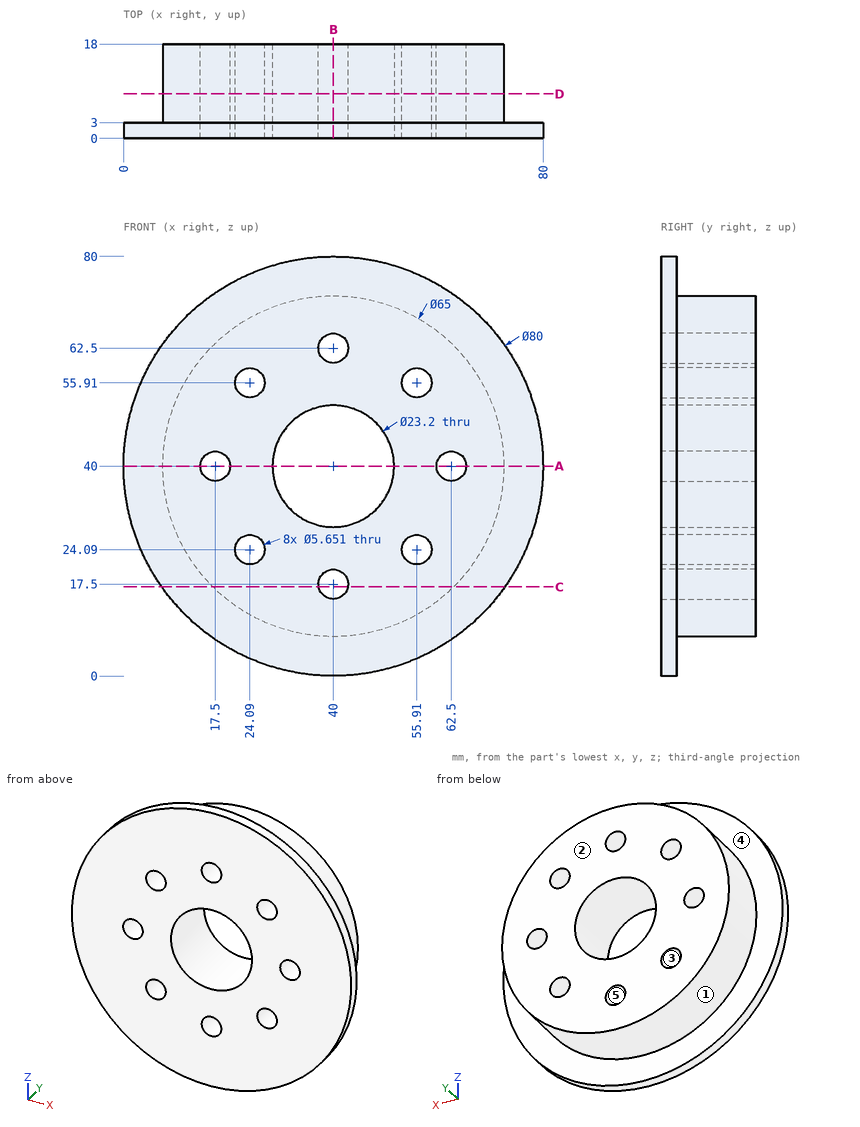
Here's the drawing with two shaded views (mm, measured from the low corner). I have some questions. A direction names the side the tool comes from. Give positions to 0.01 mm unless a question says otherwise; leave off trailing zeros. Write each loop counter-clockwise with the first axis right and the second up, starting at its lowest first coordinate (ties: lowest second). Pieces come first, ordered by that corner, then holes. Notation, with made-up numbers: (-9, 41) -> (13, 41) arc R27 cw to (13, 58) -> close; hole circle Ø4 at (27.5, 68.5). An arc over 180 degrees is marked (long way). Use one line per item in the form item = value. Start each with the question number.
1. Imagine slicing it at C-C on z = 17. List the corners of the cut face in (x, y) for me.
2. Imagine slicing it at D-D on y = 8.5. State how many separate pieces and enclosed holes the cut face has, plus the area to 4 significant figures.
3. Imagine slicing it at B-B on x = 40. List the corners of the cut face in (y, z) for me (1 decimal).
4. If I drill on L1, parallel to Z at x = 56.5, y = 3.25 (1 decimal); L2, parallel to X at y = 8.5, z = 22.5 (1 decimal), over which ranges is the centre line in solid material (lowest first)?
5. Will these pins go through, and if not, where does the flat tip stop? pin 1 Ø3 at (x, y) = (21.5, 9.5) entering from +Z; pin 2 Ø1.5 at (y, z) = (16, 65.5) entering from +X (1 decimal); pin 3 Ø10 at (x, y) = (52, 13.5) entering from -Z; pin 4 Ø4.5 at (x, z) = (55.91, 55.91) entering from -Y.
6. Imagine slicing it at A-A on z = 40. List the corners of the cut face in (x, y) for me (1 decimal), plus the area to 3 significant figures.
7. Thinking about a two-plate mould opening in Z: for the marked faces 1, 2 and 3, which applies, +Z half, -Z half, draft (parallel to the pull), parting line (faces both ways), or undercut?
8. On a 3-axis mill with a long thin cutter (end or side, diameter ignored), from which of +Z, -Z, +X, -X, +Y, -Y can I reach the whole of each face in a straight line? I mean the marked faces 4 and 5. Say none if no direction works.
Entries:
q1.outline = (7.27, 0) -> (37.22, 0) -> (37.22, 18) -> (17.04, 18) -> (17.04, 3) -> (7.27, 3) -> close; (42.78, 0) -> (72.73, 0) -> (72.73, 3) -> (62.96, 3) -> (62.96, 18) -> (42.78, 18) -> close
q2.separate_pieces = 1
q2.enclosed_holes = 9
q2.area = 2,695 mm²
q3.outline = (0, 0) -> (3, 0) -> (3, 7.5) -> (18, 7.5) -> (18, 14.7) -> (0, 14.7) -> close; (0, 20.3) -> (18, 20.3) -> (18, 28.4) -> (0, 28.4) -> close; (0, 51.6) -> (18, 51.6) -> (18, 59.7) -> (0, 59.7) -> close; (0, 65.3) -> (18, 65.3) -> (18, 72.5) -> (3, 72.5) -> (3, 80) -> (0, 80) -> close
q4.L1 = 12 to 21.3, 26.9 to 53.1, 58.7 to 68
q4.L2 = 12.6 to 21.8, 26.4 to 53.6, 58.2 to 67.4
q5.pin_1 = 67.7
q5.pin_2 = 61.1
q5.pin_3 = 8.26
q5.pin_4 = through
q6.outline = (0, 0) -> (14.7, 0) -> (14.7, 18) -> (7.5, 18) -> (7.5, 3) -> (0, 3) -> close; (20.3, 0) -> (28.4, 0) -> (28.4, 18) -> (20.3, 18) -> close; (51.6, 0) -> (59.7, 0) -> (59.7, 18) -> (51.6, 18) -> close; (65.3, 0) -> (80, 0) -> (80, 3) -> (72.5, 3) -> (72.5, 18) -> (65.3, 18) -> close
q6.area = 594 mm²
q7.face_1 = parting line
q7.face_2 = draft
q7.face_3 = undercut
q8.face_4 = +Y
q8.face_5 = +Y, -Y
